Work out the finished part from the listing and answer in its coordinate system (mm). A direction names the side the tool comes from. Round coordinates to 2 decimals unless told otherwise and drop trailing zeros. Loops run counter-clockwise (first coordinate to the right, second up) from the corner with the lowest first, then second, coordinate; pieces in that order, holes last. Notation, with made-up numbers: (-13.5, 21.5) -> (-4.5, 21.5) arc R24 ccw to (-4.5, 41.5) -> close; hole circle Ø9 at (-13, 61). An arc over 180 degrees is marked (long way). Use one line per item in the form item = value.
Autodesk Inventor part; units mm, degrees
ref_plane "Work Plane1" through (-29.1, -14.5, 2.4) normal (0, 0, -1) x (0, 1, 0)
ref_plane "Work Plane2" through (-13.8999, -10.5497, 2.25) normal (0, 0, -1) x (0, 1, 0)
ref_plane "YZ Plane" through (0, 0, 0) normal (1, 0, 0) x (0, 1, 0)
ref_plane "Work Plane1" through (-29.1, -14.5, 2.4) normal (0, 0, -1) x (0, 1, 0)
ref_plane "Work Plane2" through (-13.8999, -10.5497, 2.25) normal (0, 0, -1) x (0, 1, 0)
sketch "Sketch1" plane through (0, 0, 0) normal (0, 0, 1) x (1, 0, 0)
  line L0 (-34.86, 0) -> (34.86, 0) construction
  line L1 (0, -34.86) -> (0, 34.86) construction
  line L2 (0, 0) -> (11.1575, 11.1575) construction
  line L3 (0, 0) -> (15.7791, 0) construction
  line L4 (0, 24.9) -> (16.8009, 24.9)
  line L5 (16.8009, 24.9) -> (16.8009, 21.2415)
  line L6 (16.8009, 21.2415) -> (19.0212, 19.0212)
  line L7 (24.9, 0) -> (24.9, 16.8009)
  line L8 (24.9, 16.8009) -> (21.2415, 16.8009)
  line L9 (21.2415, 16.8009) -> (19.0212, 19.0212)
  line L10 (0, -24.9) -> (16.8009, -24.9)
  line L11 (16.8009, -24.9) -> (16.8009, -21.2415)
  line L12 (16.8009, -21.2415) -> (19.0212, -19.0212)
  line L13 (24.9, 0) -> (24.9, -16.8009)
  line L14 (24.9, -16.8009) -> (21.2415, -16.8009)
  line L15 (21.2415, -16.8009) -> (19.0212, -19.0212)
  line L16 (0, 24.9) -> (-16.8009, 24.9)
  line L17 (-16.8009, 24.9) -> (-16.8009, 21.2415)
  line L18 (-16.8009, 21.2415) -> (-19.0212, 19.0212)
  line L19 (-24.9, 16.8009) -> (-21.2415, 16.8009)
  line L20 (-21.2415, 16.8009) -> (-19.0212, 19.0212)
  line L21 (0, -24.9) -> (-16.8009, -24.9)
  line L22 (-16.8009, -24.9) -> (-16.8009, -21.2415)
  line L23 (-16.8009, -21.2415) -> (-19.0212, -19.0212)
  line L24 (-21.2415, -16.8009) -> (-19.0212, -19.0212)
  line L25 (-24.9, -16.8009) -> (-21.2415, -16.8009)
  line L26 (-24.9, 0) -> (-24.9, -16.8009)
  line L27 (-24.9, 0) -> (-24.9, 16.8009)
  circle A0 centre (0, 0) radius 5
  dimension "d0" = 45
  dimension "d2" = 24.9
  dimension "d3" = 3.14
  dimension "d4" = 26.9
  dimension "d5" = 10
extrude "Extrusion1" add sketch "Sketch1" along normal up to surface (2.25 mm away)
sketch "Sketch5" plane through (0, 0, 0) normal (0, 0, -1) x (-1, 0, 0)
  circle A0 centre (-9.7, 10) radius 1.4
  circle A1 centre (-9.7, -10) radius 1.4
  circle A2 centre (13.8, 0) radius 1.4
  circle A3 centre (-10, 6.9) radius 0.75
  circle A4 centre (10, 6.9) radius 1.25
  point P0 (0, 0)
hole "Hole1" at (9.7, -10, 0) at (9.7, 10, 0) direction (0, 0, 1) diameter 3.3 depth 12 tip angle 118
sketch "Sketch6" plane through (-16.8009, 24.9, 2.25) normal (0, 0, 1) x (1, 0, 0)
  circle A0 centre (26.5009, -34.9) radius 1.65 construction
  circle A1 centre (26.5009, -14.9) radius 1.65 construction
  circle A2 centre (16.8009, -24.9) radius 5 construction
  line L0 (33.6017, -3.6585) -> (33.6017, 0) construction
  line L1 (33.6017, 0) -> (0, 0) construction
  line L2 (0, 0) -> (0, -3.6585) construction
  line L3 (0, -3.6585) -> (-4.4406, -8.0991) construction
  line L4 (-4.4406, -8.0991) -> (-8.0991, -8.0991) construction
  line L5 (-8.0991, -8.0991) -> (-8.0991, -41.7009) construction
  line L6 (-8.0991, -41.7009) -> (-4.4406, -41.7009) construction
  line L7 (-4.4406, -41.7009) -> (0, -46.1415) construction
  line L8 (0, -46.1415) -> (0, -49.8) construction
  line L9 (0, -49.8) -> (33.6017, -49.8) construction
  line L10 (33.6017, -49.8) -> (33.6017, -46.1415) construction
  line L11 (33.6017, -46.1415) -> (38.0423, -41.7009) construction
  line L12 (38.0423, -41.7009) -> (41.7009, -41.7009) construction
  line L13 (41.7009, -41.7009) -> (41.7009, -8.0991) construction
  line L14 (41.7009, -8.0991) -> (38.0423, -8.0991) construction
  line L15 (38.0423, -8.0991) -> (33.6017, -3.6585) construction
  line L16 (33.7009, -14.9) -> (-0.0991, -14.9)
  line L17 (33.7009, -16.55) -> (-0.0991, -16.55)
  line L18 (-0.0991, -13.25) -> (33.7009, -13.25)
  arc A3 (33.7009, -16.55) -> (33.7009, -13.25) centre (33.7009, -14.9) ccw
  arc A4 (-0.0991, -13.25) -> (-0.0991, -16.55) centre (-0.0991, -14.9) ccw
  line L19 (-8.0991, -41.7009) -> (-8.0991, -8.0991) construction
  line L20 (-8.0991, -24.9) -> (41.7009, -24.9) construction
  line L21 (41.7009, -8.0991) -> (41.7009, -41.7009) construction
  circle A5 centre (26.5009, -34.9) radius 1.65 construction
  line L22 (33.7009, -34.9) -> (-0.0991, -34.9)
  line L23 (33.7009, -33.25) -> (-0.0991, -33.25)
  line L24 (-0.0991, -36.55) -> (33.7009, -36.55)
  arc A6 (33.7009, -36.55) -> (33.7009, -33.25) centre (33.7009, -34.9) ccw
  arc A7 (-0.0991, -33.25) -> (-0.0991, -36.55) centre (-0.0991, -34.9) ccw
  point P0 (16.8009, -24.9)
  point P1 (16.8009, -14.9)
  point P2 (16.8009, -34.9)
  dimension "d25" = 8
  dimension "d26" = 8
extrude "Extrusion5" cut sketch "Sketch6" against normal through all
sketch "Skizze7" plane through (-16.8009, 24.9, 2.25) normal (0, 0, 1) x (1, 0, 0)
  line L0 (33.7009, -16.55) -> (-0.0991, -16.55) construction
  arc A0 (-0.0991, -13.25) -> (-0.0991, -16.55) centre (-0.0991, -14.9) ccw construction
  line L1 (-0.0991, -13.25) -> (33.7009, -13.25) construction
  arc A1 (33.7009, -16.55) -> (33.7009, -13.25) centre (33.7009, -14.9) ccw construction
  line L2 (-0.0991, -33.25) -> (33.7009, -33.25) construction
  arc A2 (33.7009, -36.55) -> (33.7009, -33.25) centre (33.7009, -34.9) ccw construction
  line L3 (33.7009, -36.55) -> (-0.0991, -36.55) construction
  arc A3 (-0.0991, -33.25) -> (-0.0991, -36.55) centre (-0.0991, -34.9) ccw construction
  circle A4 centre (16.8009, -24.9) radius 5 construction
  line L4 (33.6017, -3.6585) -> (33.6017, 0)
  line L5 (33.6017, 0) -> (0, 0) construction
  line L6 (0, 0) -> (0, -3.6585)
  line L7 (0, -3.6585) -> (-4.4406, -8.0991)
  line L8 (-4.4406, -8.0991) -> (-8.0991, -8.0991)
  line L9 (-8.0991, -8.0991) -> (-8.0991, -41.7009) construction
  line L10 (-8.0991, -41.7009) -> (-4.4406, -41.7009)
  line L11 (-4.4406, -41.7009) -> (0, -46.1415)
  line L12 (0, -46.1415) -> (0, -49.8)
  line L13 (0, -49.8) -> (33.6017, -49.8) construction
  line L14 (33.6017, -49.8) -> (33.6017, -46.1415)
  line L15 (33.6017, -46.1415) -> (38.0423, -41.7009)
  line L16 (38.0423, -41.7009) -> (41.7009, -41.7009)
  line L17 (41.7009, -41.7009) -> (41.7009, -8.0991) construction
  line L18 (41.7009, -8.0991) -> (38.0423, -8.0991)
  line L19 (38.0423, -8.0991) -> (33.6017, -3.6585)
  line L20 (-0.1, 0.1) -> (33.7017, 0.1) construction
  line L21 (33.7017, 0.1) -> (33.7017, -3.6171)
  line L22 (33.7017, -3.6171) -> (38.0838, -7.9991)
  line L23 (38.0838, -7.9991) -> (41.8009, -7.9991)
  line L24 (41.8009, -7.9991) -> (41.8009, -41.8009) construction
  line L25 (41.8009, -41.8009) -> (38.0838, -41.8009)
  line L26 (38.0838, -41.8009) -> (33.7017, -46.1829)
  line L27 (33.7017, -46.1829) -> (33.7017, -49.9)
  line L28 (33.7017, -49.9) -> (-0.1, -49.9) construction
  line L29 (-0.1, -49.9) -> (-0.1, -46.1829)
  line L30 (-0.1, -46.1829) -> (-4.4821, -41.8009)
  line L31 (-4.4821, -41.8009) -> (-8.1991, -41.8009)
  line L32 (-8.1991, -41.8009) -> (-8.1991, -7.9991) construction
  line L33 (-8.1991, -7.9991) -> (-4.4821, -7.9991)
  line L34 (-4.4821, -7.9991) -> (-0.1, -3.6171)
  line L35 (-0.1, -3.6171) -> (-0.1, 0.1)
  line L36 (33.6017, 0) -> (0, 0)
  line L37 (0, 0) -> (-0.1, 0)
  line L38 (-8.0991, -41.7009) -> (-8.0991, -8.0991)
  line L39 (-8.0991, -8.0991) -> (-8.0991, -7.9991)
  line L40 (33.6017, 0) -> (33.6017, -3.6585)
  line L41 (33.6017, 0) -> (33.7017, 0)
  line L42 (41.7009, -8.0991) -> (41.7009, -7.9991)
  line L43 (41.7009, -41.7009) -> (38.0423, -41.7009)
  line L44 (41.7009, -41.7009) -> (41.7009, -41.8009)
  line L45 (33.6017, -49.8) -> (33.7017, -49.8)
  line L46 (0, -49.8) -> (0, -46.1415)
  line L47 (0, -49.8) -> (-0.1, -49.8)
  line L48 (-8.0991, -41.7009) -> (-8.0991, -41.8009)
  point P0 (16.8009, -24.9)
  dimension "d29" = 0.1
extrude "IM_offset" add sketch "Skizze7" against normal up to surface (2.25 mm away)
properties part number "20_Cube_insert_Sample_holder"
(1) For a pull along X with two mould halves and no side action, classify faces 1 (the flat face through (19.123, -19.061, 1.141)), 2 (the flat face through (0, -24.9, 1)), 3 (the cylindrical face through (-18.55, 10.04, 1.14)) as +X half, -X half, draft (parallel to the pull), parting line (faces both ways), or undercut.
Completed:
face_1 = +X half
face_2 = draft
face_3 = undercut
(2) Consider L1, parallel to Y at x = 7, z = 1.45; L2, parallel to Y at x = 0, z = 0.5; L3, parallel to Y at x = 4.5, z = 2.1. Determine where each line is inside the solid, lowest interval first.
Completed:
L1 = -24.9 to -11.65, -8.35 to 8.35, 11.65 to 24.9
L2 = -24.9 to -11.65, -8.35 to -5, 5 to 8.35, 11.65 to 24.9
L3 = -24.9 to -11.65, -8.35 to -2.18, 2.18 to 8.35, 11.65 to 24.9
(3) Find section C-C, the plane z = 1.85. Write down the section's boundary in (x, y).
Completed:
outline = (-24.9, -16.9) -> (-21.28, -16.9) -> (-16.9, -21.28) -> (-16.9, -24.9) -> (16.9, -24.9) -> (16.9, -21.28) -> (21.28, -16.9) -> (24.9, -16.9) -> (24.9, 16.9) -> (21.28, 16.9) -> (16.9, 21.28) -> (16.9, 24.9) -> (-16.9, 24.9) -> (-16.9, 21.28) -> (-21.28, 16.9) -> (-24.9, 16.9) -> close; hole (-16.9, -11.65) -> (16.9, -11.65) arc R1.65 ccw to (16.9, -8.35) -> (-16.9, -8.35) arc R1.65 ccw to start; hole (-16.9, 8.35) -> (16.9, 8.35) arc R1.65 ccw to (16.9, 11.65) -> (-16.9, 11.65) arc R1.65 ccw to start; hole circle Ø10 at (0, 0)
(4) For faces 4 (the flat face through (-23, -16.901, 1)), 5 (the flat face through (16.901, 23, 1)), 6 (the flat face through (0, 8.35, 1)), determine the directions among +Z, -Z, +X, -X, +Y, -Y from which every point of the face is accessible in a straight line to the end or side of a thin tool.
Completed:
face_4 = +Z, -Z, -X, -Y
face_5 = +Z, -Z, +X, +Y
face_6 = +Z, -Z
(5) Find section D-D, the plane x = -2. Write down the section's boundary in (y, z), then the cut area to 3 significant figures.
Completed:
outline = (-24.9, 0) -> (-11.65, 0) -> (-11.65, 2.25) -> (-24.9, 2.25) -> close; (-8.35, 0) -> (-4.58, 0) -> (-4.58, 2.25) -> (-8.35, 2.25) -> close; (4.58, 0) -> (8.35, 0) -> (8.35, 2.25) -> (4.58, 2.25) -> close; (11.65, 0) -> (24.9, 0) -> (24.9, 2.25) -> (11.65, 2.25) -> close
area = 76.6 mm2
(6) Find section B-B, the plane x = -11. Write down the section's boundary in (y, z), then the cut area to 3 significant figures.
Completed:
outline = (-24.9, 0) -> (-11.65, 0) -> (-11.65, 2.25) -> (-24.9, 2.25) -> close; (-8.35, 0) -> (8.35, 0) -> (8.35, 2.25) -> (-8.35, 2.25) -> close; (11.65, 0) -> (24.9, 0) -> (24.9, 2.25) -> (11.65, 2.25) -> close
area = 97.2 mm2
(7) Given P1, Ø9, axis at x = 0, y = 0, coming from the +Z side; P2, Ø5, axis at x = 13.5, y = 7.5, coming from the -Z side; P3, Ø0.7, axis at y = 23, z = 1, coming from the -X side; P4, Ø0.7, axis at x = 23, z = 1, coming from the -Y side, each flat-ended and moving along its own axis, determine where each tip first touches the part or whether it passes through.
Completed:
P1 = through
P2 = 0
P3 = -16.9
P4 = -16.9
(8) Find section A-A, the plane y = 0. Write down the section's boundary in (x, z).
Completed:
outline = (-24.9, 0) -> (-5, 0) -> (-5, 2.25) -> (-24.9, 2.25) -> close; (5, 0) -> (24.9, 0) -> (24.9, 2.25) -> (5, 2.25) -> close
